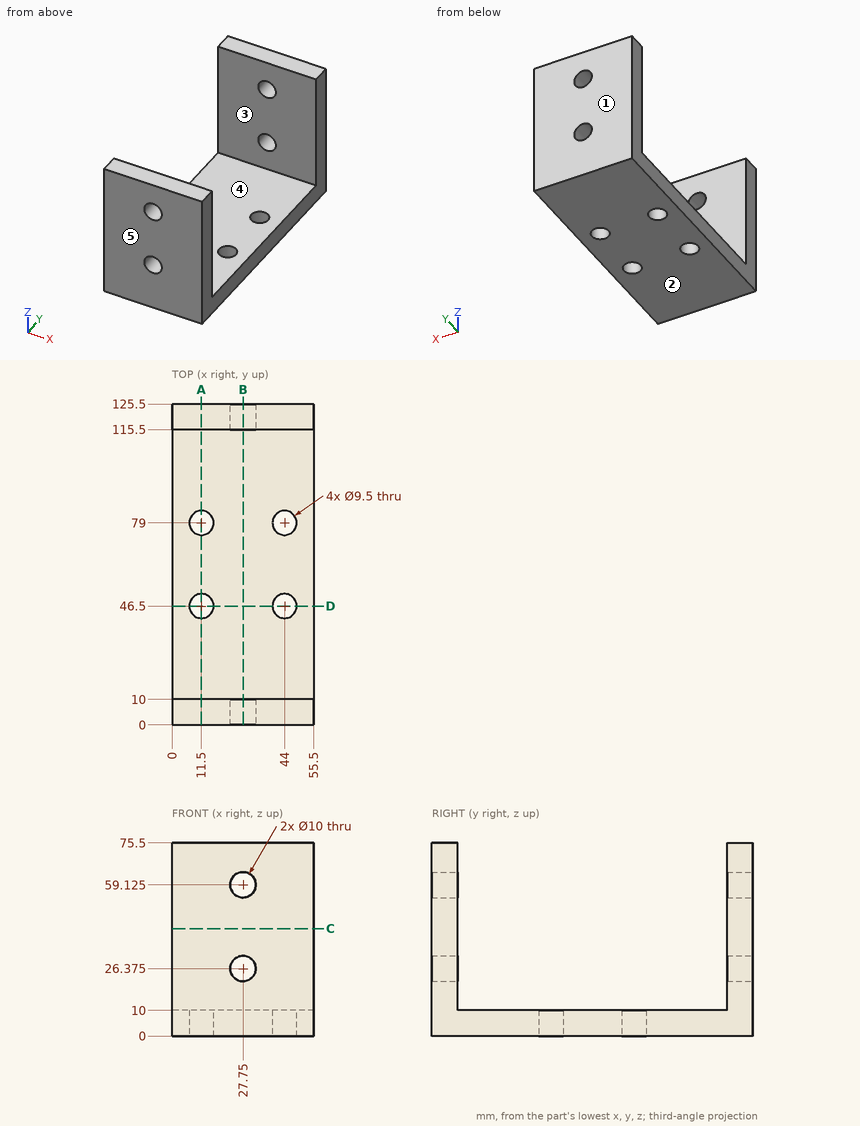
Study the drawing (mm; zero at the part's minimum x, y, z) and answer. A direction names the side the tool comes from. Coordinates: 2 decimals unless noted, no trailing zeros. Write each loop counter-clockwise with the first axis right and the second up, starting at its lowest first coordinate (ties: lowest second). Pieces come first, ordered by that corner, then holes. Notation, with made-up numbers: M 19.5,7 L 58.5,7 A31 cw 58.5,39 Z; hole C -34,-22 d6. An arc over 180 degrees is marked long. Use one line per item in the form item = value.
Item 1: Find section D-D, the plane y = 46.5. Give the vertices of the cut face in (x, z), plus the area to 3 significant figures.
Model answer:
outline = M 0,0 L 6.75,0 L 6.75,10 L 0,10 Z; M 16.25,0 L 39.25,0 L 39.25,10 L 16.25,10 Z; M 48.75,0 L 55.5,0 L 55.5,10 L 48.75,10 Z
area = 365 mm2
Item 2: Given P1, Ø11, axis at x = 11.5, y = 79, coming from the +Z side, flat-ended and moving along its own axis, determine where the tip first touches the part or whether it passes through.
Model answer:
P1 = 10
Item 3: Find the intervals of material crossed by probe 1 along Z at (x, y) = (27.75, 6) (3 decimals); probe 2 along Y at (x, z) = (49.5, 61); probe 3 along X at (y, z) = (46, 2), in increasing order.
Model answer:
probe_1 = 0 to 21.375, 31.375 to 54.125, 64.125 to 75.5
probe_2 = 0 to 10, 115.5 to 125.5
probe_3 = 0 to 6.78, 16.22 to 39.28, 48.72 to 55.5
Item 4: Find section B-B, the plane x = 27.75. Give the vertices of the cut face in (y, z) (3 decimals), plus the area to 4 significant figures.
Model answer:
outline = M 0,0 L 125.5,0 L 125.5,21.375 L 115.5,21.375 L 115.5,10 L 10,10 L 10,21.375 L 0,21.375 Z; M 0,31.375 L 10,31.375 L 10,54.125 L 0,54.125 Z; M 0,64.125 L 10,64.125 L 10,75.5 L 0,75.5 Z; M 115.5,31.375 L 125.5,31.375 L 125.5,54.125 L 115.5,54.125 Z; M 115.5,64.125 L 125.5,64.125 L 125.5,75.5 L 115.5,75.5 Z
area = 2,165 mm2
Item 5: The mould has two halves that part along Y. Classify the marked faces 1, 2 and 3: released by +Y, released by -Y, zero draft, split by the parting line, or undercut.
Model answer:
face_1 = released by +Y
face_2 = zero draft
face_3 = undercut
Item 6: For the marked faces 4 and 5, determine the directions among +Z, -Z, +X, -X, +Y, -Y from which every point of the face is accessible in a straight line to the end or side of a thin tool.
Model answer:
face_4 = +Z, +X, -X
face_5 = +Z, -Z, +X, -X, -Y
Item 7: Find section C-C, the plane z = 42. Give the vertices of the cut face in (x, y).
Model answer:
outline = M 0,0 L 55.5,0 L 55.5,10 L 0,10 Z; M 0,115.5 L 55.5,115.5 L 55.5,125.5 L 0,125.5 Z
Item 8: Find section A-A, the plane x = 11.5. Give the vertices of the cut face in (y, z).
Model answer:
outline = M 0,0 L 41.75,0 L 41.75,10 L 10,10 L 10,75.5 L 0,75.5 Z; M 51.25,0 L 74.25,0 L 74.25,10 L 51.25,10 Z; M 83.75,0 L 125.5,0 L 125.5,75.5 L 115.5,75.5 L 115.5,10 L 83.75,10 Z
